Geometry: final body of the model. Coordinates: model frame, mm. Give positions to 0.01 mm unless a question says otherwise; leave off trailing zeros. Write each loop counter-clockwise with the first axis right and the second up, starting at its lowest first coordinate (ties: lowest second). Pieces come first, ordered by that corner, then holes. Notation, with made-up numbers: M -16.5,47 L 20.5,47 A31 cw 20.5,80 Z; hole C 59,80.5 d5. An arc over 180 degrees is marked long. Use one line per item in the form item = value. Start each with the question number.
Item 1: Section query A-A on x = 71. Return loops of the section in (y, z), then the cut area to 3 significant figures.
Item 2: Section query C-C on y = 1.7. Give the number of separate pieces and of enclosed holes in the cut face, then the cut area to 3 significant figures.
Item 3: Contact query for flat-ended pins moving along their axis: P1, Ø1.5, axis at x = 24.5, y = 1, coming from the +Z side; P2, Ø2.5, axis at x = 185, z = -200.5, coming from the +Y side; P3, Ø0.9, axis at y = 1, z = -266.5, coming from the -X side; P4, Ø0.9, axis at x = 68, y = 2, coming from the +Z side. Output: stop coordinate, or through.
Item 4: Section query B-B on z = -78. Return loops of the section in (x, y).
Item 5: Section query D-D on z = -194. Return loops of the section in (x, y), then the cut area to 3 significant figures.
Item 6: Material intervals for line 1 along X through (y, z) = (0.8, -247); line 2 along Z through (x, y) = (86, 0.7); line 3 along X through (y, z) = (1, -104.5), sorted ascending. Write a range as from..to.
from build123d import *

# Parameters (mm, degrees)
CROQUIS1_W              = 220
CROQUIS1_H              = 320
CROQUIS1_R              = 1.7
CROQUIS1_R_2            = 1.6
SALIENTE_EXTRUIR1_DEPTH = 3
CROQUIS2_OUTSIDE_W      = 299.668
CROQUIS2_OUTSIDE_H      = 399.668
CORTAR_EXTRUIR1_DEPTH   = 3
REDONDEO1_R             = 5
CROQUIS4_W              = 15
CROQUIS4_H              = 60
CORTAR_EXTRUIR3_DEPTH   = 3


with BuildPart() as part:
    # Croquis1 → Saliente-Extruir1 (new body)
    with BuildSketch(Plane(origin=(0, 0, 0), x_dir=(1, 0, 0), z_dir=(0, 1, 0))):
        with Locations((110, 160)):
            Rectangle(CROQUIS1_W, CROQUIS1_H)
        with Locations(Location((35, 215.5, 0), (0, 0, 270))):
            Circle(CROQUIS1_R, mode=Mode.SUBTRACT)
        with Locations(Location((35, 200.5, 0), (0, 0, 270))):
            Circle(CROQUIS1_R, mode=Mode.SUBTRACT)
        with Locations(Location((35, 119.5, 0), (0, 0, 90))):
            Circle(CROQUIS1_R, mode=Mode.SUBTRACT)
        with Locations(Location((35, 104.5, 0), (0, 0, 90))):
            Circle(CROQUIS1_R, mode=Mode.SUBTRACT)
        with Locations(Location((5.5, 314.5, 0), (0, 0, 270))):
            Circle(CROQUIS1_R_2, mode=Mode.SUBTRACT)
        with Locations(Location((214.5, 314.5, 0), (0, 0, 90))):
            Circle(CROQUIS1_R_2, mode=Mode.SUBTRACT)
        with Locations(Location((214.5, 5.5, 0), (0, 0, 270))):
            Circle(CROQUIS1_R_2, mode=Mode.SUBTRACT)
        with Locations(Location((5.5, 5.5, 0), (0, 0, 90))):
            Circle(CROQUIS1_R_2, mode=Mode.SUBTRACT)
        with Locations(Location((15, 200.5, 0), (0, 0, 90))):
            Circle(CROQUIS1_R, mode=Mode.SUBTRACT)
        with Locations(Location((15, 215.5, 0), (0, 0, 90))):
            Circle(CROQUIS1_R, mode=Mode.SUBTRACT)
        with Locations(Location((15, 104.5, 0), (0, 0, 270))):
            Circle(CROQUIS1_R, mode=Mode.SUBTRACT)
        with Locations(Location((15, 119.5, 0), (0, 0, 270))):
            Circle(CROQUIS1_R, mode=Mode.SUBTRACT)
        with Locations(Location((110, 180, 0), (0, 0, 270))):
            Circle(CROQUIS1_R_2, mode=Mode.SUBTRACT)
        with Locations(Location((110, 140, 0), (0, 0, 90))):
            Circle(CROQUIS1_R_2, mode=Mode.SUBTRACT)
        with Locations(Location((5.5, 160, 0), (0, 0, 270))):
            Circle(CROQUIS1_R_2, mode=Mode.SUBTRACT)
        with Locations(Location((214.5, 160, 0), (0, 0, 90))):
            Circle(CROQUIS1_R_2, mode=Mode.SUBTRACT)
        with Locations(Location((185, 104.5, 0), (0, 0, 270))):
            Circle(CROQUIS1_R, mode=Mode.SUBTRACT)
        with Locations(Location((185, 119.5, 0), (0, 0, 270))):
            Circle(CROQUIS1_R, mode=Mode.SUBTRACT)
        with Locations(Location((205, 119.5, 0), (0, 0, 90))):
            Circle(CROQUIS1_R, mode=Mode.SUBTRACT)
        with Locations(Location((205, 104.5, 0), (0, 0, 90))):
            Circle(CROQUIS1_R, mode=Mode.SUBTRACT)
        with Locations(Location((185, 215.5, 0), (0, 0, 90))):
            Circle(CROQUIS1_R, mode=Mode.SUBTRACT)
        with Locations(Location((185, 200.5, 0), (0, 0, 90))):
            Circle(CROQUIS1_R, mode=Mode.SUBTRACT)
        with Locations(Location((205, 200.5, 0), (0, 0, 270))):
            Circle(CROQUIS1_R, mode=Mode.SUBTRACT)
        with Locations(Location((205, 215.5, 0), (0, 0, 270))):
            Circle(CROQUIS1_R, mode=Mode.SUBTRACT)
    extrude(amount=SALIENTE_EXTRUIR1_DEPTH)

    # Croquis2 outside → Cortar-Extruir1 (cut)
    # profile 1 of 9: a face of its own
    with BuildSketch(Plane(origin=(0, 3, 0), x_dir=(1, 0, 0), z_dir=(0, 1, 0))):
        with Locations((110, 160)):
            Rectangle(CROQUIS2_OUTSIDE_W, CROQUIS2_OUTSIDE_H)
        with BuildLine():
            Line((9, 148.77502784), (9, 94.5))
            Line((9, 94.5), (19, 94.5))
            Line((19, 94.5), (19, 30))
            Line((19, 30), (1.298802547, 9.049639413))
            ThreePointArc((1.298802547, 9.049639413), (1.950360587, 1.298802547), (9.701197453, 1.950360587))
            Line((9.701197453, 1.950360587), (24.106631311, 19))
            Line((24.106631311, 19), (195.893368689, 19))
            Line((195.893368689, 19), (210.298802547, 1.950360587))
            ThreePointArc((210.298802547, 1.950360587), (218.049639413, 1.298802547), (218.701197453, 9.049639413))
            Line((218.701197453, 9.049639413), (201, 30))
            Line((201, 30), (201, 94.5))
            Line((201, 94.5), (211, 94.5))
            Line((211, 94.5), (211, 148.77502784))
            ThreePointArc((211, 148.77502784), (212.318863014, 152.528287293), (215.695652174, 154.631535054))
            ThreePointArc((215.695652174, 154.631535054), (220, 160), (215.695652174, 165.368464946))
            ThreePointArc((215.695652174, 165.368464946), (212.318863014, 167.471712707), (211, 171.22497216))
            Line((211, 171.22497216), (211, 225.5))
            Line((211, 225.5), (201, 225.5))
            Line((201, 225.5), (201, 290))
            Line((201, 290), (218.701197453, 310.950360587))
            ThreePointArc((218.701197453, 310.950360587), (218.049639413, 318.701197453), (210.298802547, 318.049639413))
            Line((210.298802547, 318.049639413), (195.893368689, 301))
            Line((195.893368689, 301), (24.106631311, 301))
            Line((24.106631311, 301), (9.701197453, 318.049639413))
            ThreePointArc((9.701197453, 318.049639413), (1.950360587, 318.701197453), (1.298802547, 310.950360587))
            Line((1.298802547, 310.950360587), (19, 290))
            Line((19, 290), (19, 225.5))
            Line((19, 225.5), (9, 225.5))
            Line((9, 225.5), (9, 171.22497216))
            ThreePointArc((9, 171.22497216), (7.681136986, 167.471712707), (4.304347826, 165.368464946))
            ThreePointArc((4.304347826, 165.368464946), (0, 160), (4.304347826, 154.631535054))
            ThreePointArc((4.304347826, 154.631535054), (7.681136986, 152.528287293), (9, 148.77502784))
        make_face(mode=Mode.SUBTRACT)
    # profile 2 of 9: a face of its own
    with BuildSketch(Plane(origin=(0, 3, 0), x_dir=(1, 0, 0), z_dir=(0, 1, 0))):
        with BuildLine():
            Line((182, 276), (182, 236))
            ThreePointArc((182, 236), (179.071067812, 228.928932188), (172, 226))
            Line((172, 226), (118, 226))
            ThreePointArc((118, 226), (116.585786438, 226.585786438), (116, 228))
            Line((116, 228), (116, 284))
            ThreePointArc((116, 284), (116.585786438, 285.414213562), (118, 286))
            Line((118, 286), (172, 286))
            ThreePointArc((172, 286), (179.071067812, 283.071067812), (182, 276))
        make_face()
    # profile 3 of 9: a face of its own
    with BuildSketch(Plane(origin=(0, 3, 0), x_dir=(1, 0, 0), z_dir=(0, 1, 0))):
        with BuildLine():
            Line((102, 286), (48, 286))
            ThreePointArc((48, 286), (40.928932188, 283.071067812), (38, 276))
            Line((38, 276), (38, 236))
            ThreePointArc((38, 236), (40.928932188, 228.928932188), (48, 226))
            Line((48, 226), (102, 226))
            ThreePointArc((102, 226), (103.414213562, 226.585786438), (104, 228))
            Line((104, 228), (104, 284))
            ThreePointArc((104, 284), (103.414213562, 285.414213562), (102, 286))
        make_face()
    # profile 4 of 9: a face of its own
    with BuildSketch(Plane(origin=(0, 3, 0), x_dir=(1, 0, 0), z_dir=(0, 1, 0))):
        with BuildLine():
            Line((102, 94), (48, 94))
            ThreePointArc((48, 94), (40.928932188, 91.071067812), (38, 84))
            Line((38, 84), (38, 44))
            ThreePointArc((38, 44), (40.928932188, 36.928932188), (48, 34))
            Line((48, 34), (102, 34))
            ThreePointArc((102, 34), (103.414213562, 34.585786438), (104, 36))
            Line((104, 36), (104, 92))
            ThreePointArc((104, 92), (103.414213562, 93.414213562), (102, 94))
        make_face()
    # profile 5 of 9: a face of its own
    with BuildSketch(Plane(origin=(0, 3, 0), x_dir=(1, 0, 0), z_dir=(0, 1, 0))):
        with BuildLine():
            Line((116, 36), (116, 92))
            ThreePointArc((116, 92), (116.585786438, 93.414213562), (118, 94))
            Line((118, 94), (172, 94))
            ThreePointArc((172, 94), (179.071067812, 91.071067812), (182, 84))
            Line((182, 84), (182, 44))
            ThreePointArc((182, 44), (179.071067812, 36.928932188), (172, 34))
            Line((172, 34), (118, 34))
            ThreePointArc((118, 34), (116.585786438, 34.585786438), (116, 36))
        make_face()
    # profile 6 of 9: a face of its own
    with BuildSketch(Plane(origin=(0, 3, 0), x_dir=(1, 0, 0), z_dir=(0, 1, 0))):
        with BuildLine():
            Line((45, 152), (45, 119))
            ThreePointArc((45, 119), (47.928932188, 111.928932188), (55, 109))
            Line((55, 109), (85, 109))
            ThreePointArc((85, 109), (92.071067812, 111.928932188), (95, 119))
            Line((95, 119), (95, 152))
            ThreePointArc((95, 152), (94.414213562, 153.414213562), (93, 154))
            Line((93, 154), (47, 154))
            ThreePointArc((47, 154), (45.585786438, 153.414213562), (45, 152))
        make_face()
    # profile 7 of 9: a face of its own
    with BuildSketch(Plane(origin=(0, 3, 0), x_dir=(1, 0, 0), z_dir=(0, 1, 0))):
        with BuildLine():
            Line((93, 166), (47, 166))
            ThreePointArc((47, 166), (45.585786438, 166.585786438), (45, 168))
            Line((45, 168), (45, 201))
            ThreePointArc((45, 201), (47.928932188, 208.071067812), (55, 211))
            Line((55, 211), (85, 211))
            ThreePointArc((85, 211), (92.071067812, 208.071067812), (95, 201))
            Line((95, 201), (95, 168))
            ThreePointArc((95, 168), (94.414213562, 166.585786438), (93, 166))
        make_face()
    # profile 8 of 9: a face of its own
    with BuildSketch(Plane(origin=(0, 3, 0), x_dir=(1, 0, 0), z_dir=(0, 1, 0))):
        with BuildLine():
            Line((135, 109), (165, 109))
            ThreePointArc((165, 109), (172.071067812, 111.928932188), (175, 119))
            Line((175, 119), (175, 152))
            ThreePointArc((175, 152), (174.414213562, 153.414213562), (173, 154))
            Line((173, 154), (127, 154))
            ThreePointArc((127, 154), (125.585786438, 153.414213562), (125, 152))
            Line((125, 152), (125, 119))
            ThreePointArc((125, 119), (127.928932188, 111.928932188), (135, 109))
        make_face()
    # profile 9 of 9: a face of its own
    with BuildSketch(Plane(origin=(0, 3, 0), x_dir=(1, 0, 0), z_dir=(0, 1, 0))):
        with BuildLine():
            Line((127, 166), (173, 166))
            ThreePointArc((173, 166), (174.414213562, 166.585786438), (175, 168))
            Line((175, 168), (175, 201))
            ThreePointArc((175, 201), (172.071067812, 208.071067812), (165, 211))
            Line((165, 211), (135, 211))
            ThreePointArc((135, 211), (127.928932188, 208.071067812), (125, 201))
            Line((125, 201), (125, 168))
            ThreePointArc((125, 168), (125.585786438, 166.585786438), (127, 166))
        make_face()
    extrude(amount=-CORTAR_EXTRUIR1_DEPTH, mode=Mode.SUBTRACT)

    # Redondeo1
    redondeo1_edges = [part.edges().sort_by_distance(p)[0] for p in [
        (211, 1.5, -225.5),
        (211, 1.5, -94.5),
        (9, 1.5, -225.5),
        (9, 1.5, -94.5),
        (24.106631311, 1.5, -301),
        (195.893368689, 1.5, -301),
        (201, 1.5, -290),
        (201, 1.5, -225.5),
        (201, 1.5, -94.5),
        (201, 1.5, -30),
        (195.893368689, 1.5, -19),
        (24.106631311, 1.5, -19),
        (19, 1.5, -30),
        (19, 1.5, -94.5),
        (19, 1.5, -290),
        (19, 1.5, -225.5),
    ]]
    fillet(redondeo1_edges, radius=REDONDEO1_R - 0.0001)  # a hair under: the kernel refuses the full size

    # Croquis4 → Cortar-Extruir3 (cut)
    with BuildSketch(Plane(origin=(0, 3, 0), x_dir=(1, 0, 0), z_dir=(0, 1, 0))):
        with Locations((24.5, 160)):
            Rectangle(CROQUIS4_W, CROQUIS4_H)
        with Locations((195.5, 160)):
            Rectangle(CROQUIS4_W, CROQUIS4_H)
    extrude(amount=-CORTAR_EXTRUIR3_DEPTH, mode=Mode.SUBTRACT)


solid = part.part
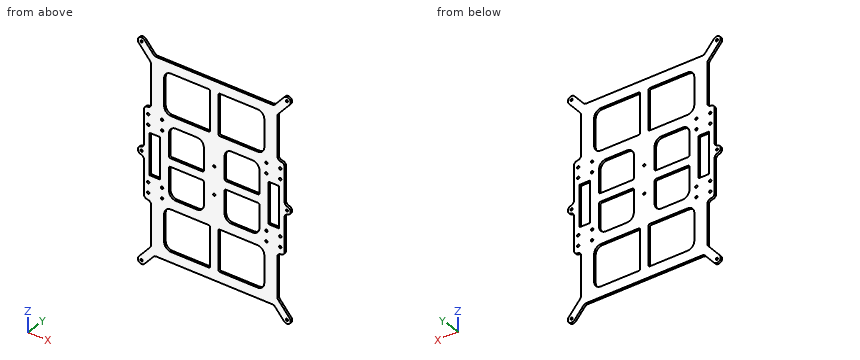
Answer sheet:
q1.outline = M 0,-301 L 3,-301 L 3,-286 L 0,-286 Z; M 0,-226 L 3,-226 L 3,-211 L 0,-211 Z; M 0,-166 L 3,-166 L 3,-154 L 0,-154 Z; M 0,-109 L 3,-109 L 3,-94 L 0,-94 Z; M 0,-34 L 3,-34 L 3,-19 L 0,-19 Z
q1.area = 216 mm2
q2.separate_pieces = 1
q2.enclosed_holes = 34
q2.area = 28,800 mm2
q3.P1 = -18.22
q3.P2 = through
q3.P3 = 19
q3.P4 = -19
q4.outline = M 19,0 L 38,0 L 38,3 L 19,3 Z; M 104,0 L 116,0 L 116,3 L 104,3 Z; M 182,0 L 201,0 L 201,3 L 182,3 Z
q5.outline = M 9,0 L 45,0 L 45,3 L 9,3 Z; M 95,0 L 125,0 L 125,3 L 95,3 Z; M 175,0 L 211,0 L 211,3 L 175,3 Z
q5.area = 306 mm2
q6.line_1 = 19..38, 104..116, 182..201
q6.line_2 = -301..-286, -226..-210.95, -166..-154, -109.05..-94, -34..-19
q6.line_3 = 9..13.3, 16.7..33.3, 36.7..183.3, 186.7..203.3, 206.7..211
